from build123d import *

# Parameters (mm, degrees)
F1_DEPTH = 25
F2_R     = 5
F3_R     = 5
F4_DEPTH = 42.9
F5_R     = 10


# Not quite as in the source:
# - a feature names something its author has since deleted; it is built from what else it names


with BuildPart() as f1:
    # F0 (on Front) → F1 (new body)
    with BuildSketch(Plane.XZ):
        with BuildLine():
            ThreePointArc((-13.2998284399, -21.1687166231), (0, 25), (13.2998284399, -21.1687166231))
            Line((13.2998284399, -21.1687166231), (13.2998284399, -46.1687166231))
            Line((13.2998284399, -46.1687166231), (16.2998284399, -46.1687166231))
            Line((16.2998284399, -46.1687166231), (16.2998284399, -22.7665454742))
            ThreePointArc((16.2998284399, -22.7665454742), (0, 28), (-16.2998284399, -22.7665454742))
            Line((-16.2998284399, -22.7665454742), (-16.2998284399, -46.2509857135))
            Line((-16.2998284399, -46.2509857135), (-13.2998284399, -46.2509857135))
            Line((-13.2998284399, -46.2509857135), (-13.2998284399, -21.1687166231))
        make_face()
    extrude(amount=F1_DEPTH)

    # F2
    f2_edges = [f1.edges().sort_by_distance(p)[0] for p in [
        (13.299828, -12.5, -21.168717),
        (-13.299828, -12.5, -21.168717),
    ]]
    fillet(f2_edges, radius=F2_R)

    # F3 (on face) → F4 (cut)
    with BuildSketch(Plane(origin=(-16.2998284399, 0, 0), x_dir=(0, -1, 0), z_dir=(-1, 0, 0))):
        with Locations((12.3893171549, -37.9563570023)):
            Circle(F3_R)
    extrude(amount=-F4_DEPTH, mode=Mode.SUBTRACT)

    # F5
    f5_edges = [f1.edges().sort_by_distance(p)[0] for p in [
        (-14.799828, 0, -46.250986),
        (-14.799828, -25, -46.250986),
        (14.799828, -25, -46.168717),
        (14.799828, 0, -46.168717),
    ]]
    fillet(f5_edges, radius=F5_R)


solid = f1.part
Could you check a few things on this model? Use its own coordinates, in mm. A direction names the side the tool comes from. Give positions to 0.01 mm unless a question says otherwise; leave off trailing zeros. Loops run counter-clockwise (first coordinate to the right, second up) from the corner with the lowest first, then second, coordinate; pieces in that order, holes last. Notation, with made-up numbers: M 6.5,-20.75 L 64.5,-20.75 A24 ccw 64.5,5.25 Z; hole C 19,-36.75 d6. An arc over 180 degrees is marked long. Answer as a JSON object with one key per item and string values.
Q1. For P1, Ø11.5, axis at y = -12.39, z = -37.96, coming from the +X side; P2, Ø2, axis at x = 1, y = -19, coming from the -Z side; P3, Ø8, axis at y = -3.5, z = -8, coming from the -X side; P4, Ø3, axis at x = -20, z = -8, coming from the +Y side, each with a flat end and sliding along its axis, tell me the tip position at first contact or that it passes through.
Values found:
{"P1": "stops at x = 16.3", "P2": "stops at z = 24.92", "P3": "stops at x = -27.71", "P4": "passes through"}
Q2. Suppose I cut it at A-A, the plane z = 0. List the corners of the cut face in (x, y) for me, plus the area to 3 significant figures.
Values found:
{"outline": "M -28,-25 L -25,-25 L -25,0 L -28,0 Z; M 25,-25 L 28,-25 L 28,0 L 25,0 Z", "area": "150 mm²"}
Q3. If I drill on probe 1 along X at (y, z) = (-6.5, -39); probe 2 along Z at (x, y) = (16, -17); probe 3 along X at (y, z) = (-0.75, 21.5), over which ranges is the centre line in solid material (lowest first)? Write a range as [from, to].
Values found:
{"probe 1": "x = [-16.3, -13.3], [13.3, 16.3]", "probe 2": "z = [-45.97, -39.89], [-36.02, -19.21], [19.21, 22.98]", "probe 3": "x = [-17.94, -12.76], [12.76, 17.94]"}
Q4. Suppose I cut it at D-D, the plane x = 0. List the corners of the cut face in (y, z) for me, plus the area to 3 significant figures.
Values found:
{"outline": "M -25,25 L 0,25 L 0,28 L -25,28 Z", "area": "75.0 mm²"}
Q5. Suppose I cut it at C-C, the plane y = -19.25. List the corners of the cut face in (x, z) for me, plus the area to 3 significant figures.
Values found:
{"outline": "M -16.3,-45.3 L -13.3,-45.3 L -13.3,-23.77 A5 ccw -15.25,-19.81 A25 cw long 15.25,-19.81 A5 ccw 13.3,-23.77 L 13.3,-45.22 L 16.3,-45.22 L 16.3,-22.77 A28 ccw long -16.3,-22.77 Z", "area": "543 mm²"}
Q6. If we mould it in two halves opening along Z, with no side actions, what happens to faces 6 (the flat face through (13.3, -12, -32)), 7 (the cylindrical face through (-0.87, -12.325, 24.985)), 8 (the cylindrical face through (14.82, -22.15, -43.16)), 9 (the cylindrical face through (13.828, -12.675, -21.536))? For each: pulls with the +Z half, pulls with the -Z half, needs draft (parallel to the pull), parting line crosses it, or undercut.
Values found:
{"face 6": "needs draft", "face 7": "undercut", "face 8": "pulls with the -Z half", "face 9": "undercut"}
Q7. Suppose I cut it at B-B, the plane y = -13.25. List the corners of the cut face in (x, z) for me, plus the area to 3 significant figures.
Values found:
{"outline": "M -16.3,-46.25 L -13.3,-46.25 L -13.3,-42.88 L -16.3,-42.88 Z; M -16.3,-33.03 L -13.3,-33.03 L -13.3,-23.77 A5 ccw -15.25,-19.81 A25 cw long 15.25,-19.81 A5 ccw 13.3,-23.77 L 13.3,-33.03 L 16.3,-33.03 L 16.3,-22.77 A28 ccw long -16.3,-22.77 Z; M 13.3,-46.17 L 16.3,-46.17 L 16.3,-42.88 L 13.3,-42.88 Z", "area": "490 mm²"}
Q8. For faces 1 (the cylindrical face through (14.82, -2.85, -43.16)), 2 (the flat face through (-16.3, -12, -32)), 3 (the cylindrical face through (-13.828, -12.675, -21.536)), 4 (the flat face through (-13.3, -12.3, -32.7)), 5 (the flat face through (16.3, -12, -32)), which set-ups out of +Z, -Z, +X, -X, +Y, -Y let a thin tool reach every point of the face, with its end or its side?
Values found:
{"face 1": "-Z, +X, +Y", "face 2": "-Z, -X, +Y, -Y", "face 3": "+Y, -Y", "face 4": "-Z, +Y, -Y", "face 5": "-Z, +X, +Y, -Y"}
